```python
from build123d import *

# Parameters (mm, degrees)
SKETCH1_W           = 32.5
SKETCH1_H           = 33
BOSS_EXTRUDE1_DEPTH = 4
SKETCH2_W           = 10
SKETCH2_H           = 4
SKETCH2_W_2         = 4
SKETCH2_H_2         = 10
BOSS_EXTRUDE2_DEPTH = 4


with BuildPart() as part:
    # Sketch1 → Boss-Extrude1 (new body)
    with BuildSketch(Plane(origin=(0, 0, 0), x_dir=(1, 0, 0), z_dir=(0, 1, 0))):
        with Locations((16.25, -16.5)):
            Rectangle(SKETCH1_W, SKETCH1_H)
    extrude(amount=BOSS_EXTRUDE1_DEPTH)

    # Sketch2 → Boss-Extrude2 (add, through all)
    with BuildSketch(Plane.XZ):
        with Locations((16.25, 35)):
            Rectangle(SKETCH2_W, SKETCH2_H)
        with Locations((34.5, 16)):
            Rectangle(SKETCH2_W_2, SKETCH2_H_2)
        with Locations((-2, 16)):
            Rectangle(SKETCH2_W_2, SKETCH2_H_2)
    extrude(amount=-BOSS_EXTRUDE2_DEPTH)


solid = part.part
```
Can you work these out from the model? Positions are in its coordinate system, mm. A direction names the side the tool comes from. Coordinates: 2 decimals unless noted, no trailing zeros. Loops run counter-clockwise (first coordinate to the right, second up) from the corner with the lowest first, then second, coordinate; pieces in that order, holes last.
Item 1: I'm going to push flat-ended pins straight in: pin 1 (2 mm diameter, centred on x = 35, y = 1, fed in from -Z); pin 2 (1.2 mm diameter, centred on y = 3, z = 35.5, fed in from -X); pin 3 (2 mm diameter, centred on y = 3, z = 28.5, fed in from +X). Where does each tip first touch, or does it pass through?
Answers below:
pin 1: stops at z = 11
pin 2: stops at x = 11.25
pin 3: stops at x = 32.5
Item 2: Suppose I cut it at A-A (y = 2.9). Please give me the cut outline in (x, z), then the cut area to 3 significant figures.
Answers below:
outline: (-4, 11) - (0, 11) - (0, 0) - (32.5, 0) - (32.5, 11) - (36.5, 11) - (36.5, 21) - (32.5, 21) - (32.5, 33) - (21.25, 33) - (21.25, 37) - (11.25, 37) - (11.25, 33) - (0, 33) - (0, 21) - (-4, 21) - close
area: 1,190 mm2
Item 3: Suppose I cut it at C-C (x = 7). Please give me the cut outline in (y, z), then the cut area to 3 significant figures.
Answers below:
outline: (0, 0) - (4, 0) - (4, 33) - (0, 33) - close
area: 132 mm2
Item 4: Suppose I cut it at B-B (z = 27). Please give me the cut outline in (x, y).
Answers below:
outline: (0, 0) - (32.5, 0) - (32.5, 4) - (0, 4) - close
Item 5: Please list where these lines run through material, in increasing order: L1, parallel to X at y = 0.35, z = 32; L2, parallel to Z at x = 10, y = 2.3; L3, parallel to Z at x = -2, y = 3.7.
Answers below:
L1: x = 0 to 32.5
L2: z = 0 to 33
L3: z = 11 to 21
Item 6: Which directions (+Z, -Z, +X, -X, +Y, -Y) give clear straight access to the entire face, cutting with the end or side of a thin tool? Please do faces 1 (the face through (34, 2, 21)), 2 (the face through (-2, 2, 21)), 3 (the face through (0, 2, 6)), 4 (the face through (32.5, 2, 6)).
Answers below:
face 1: +Z, +X, +Y, -Y
face 2: +Z, -X, +Y, -Y
face 3: -Z, -X, +Y, -Y
face 4: -Z, +X, +Y, -Y
